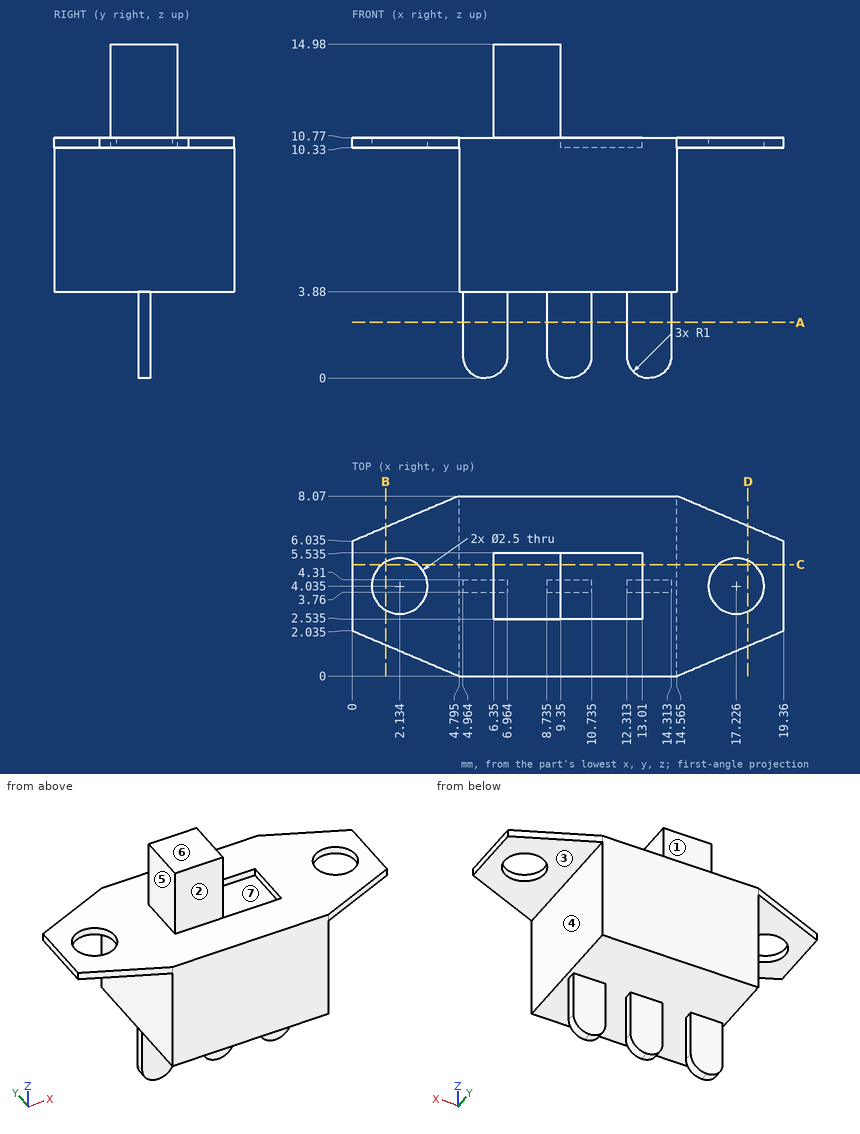
Verification items for this drawing (mm, ordinates from the low corner). A direction names the side the tool comes from. Round coordinates to 2 decimals unless told otherwise and drop trailing zeros. Write each loop counter-clockwise with the first axis right and the second up, starting at its lowest first coordinate (ties: lowest second). Pieces come first, ordered by that corner, then holes. Notation, with made-up numbers: (-20.75, 4.25) - (-4.75, 4.25) arc R31 ccw to (-4.75, 42.25) - close; hole circle Ø11 at (9, -19.75). An arc over 180 degrees is marked (long way). Answer as a JSON object with one key per item and string values. Group by question number.
Q1. Tool access check on the marked faces 1, 2 and 3. Record the directions out of +Z, -Z, +X, -X, +Y, -Y that give a thin tool (end or side, any length) a straight path to the whole face; none if there is none.
Q2. Thickness scan on line 1 (X direction, y = 2, z = 6.25) (1 decimal); line 2 (Z direction, x = 13.5, y = 0.75); line 3 (Z direction, x = 15.25, y = 3). Record the ranges inside material, lowest first.
Q3. Mould release check, pull along X, two halves, no side actions. Record for the marked faces 4, 5, 6 and 7: released by +X, released by -X, zero draft, split by the parting line, or undercut.
Q4. Go/stop test with flat-tipped pins: pin 1 Ø4 at (y, z) = (7, 8) entering from -X (1 decimal); pin 2 Ø3.5 at (x, y) = (12, 4.5) entering from +Z; pin 3 Ø1.6 at (x, z) = (14, 2) entering from +Y. Record where each tip stops, or that it passes through.
Q5. Section check A-A, the plane z = 2.5. Enter the section's corners in (x, y) (1 decimal).
Q6. Section check B-B, the plane x = 1.5. Enter the section's corners in (y, z).
Q7. Section check C-C, the plane y = 5. Give the number of separate pieces and of enclosed holes in the cut face.
Q8. Section check D-D, the plane x = 17.75. Enter the section's corners in (y, z).
Found:
{
 "1": {"face 1": "+Z, +X, -X, +Y", "face 2": "+Z, +X, -X, -Y", "face 3": "-Z, +X, +Y, -Y"},
 "2": {"line 1": "x = 4.8 to 14.6", "line 2": "z = 3.88 to 10.77", "line 3": "z = 10.33 to 10.77"},
 "3": {"face 4": "released by +X", "face 5": "released by -X", "face 6": "zero draft", "face 7": "undercut"},
 "4": {"pin 1": "stops at x = 4.8", "pin 2": "stops at z = 10.77", "pin 3": "stops at y = 4.31"},
 "5": {"outline": "(5, 3.8) - (7, 3.8) - (7, 4.3) - (5, 4.3) - close; (8.7, 3.8) - (10.7, 3.8) - (10.7, 4.3) - (8.7, 4.3) - close; (12.3, 3.8) - (14.3, 3.8) - (14.3, 4.3) - (12.3, 4.3) - close"},
 "6": {"outline": "(1.4, 10.33) - (2.96, 10.33) - (2.96, 10.77) - (1.4, 10.77) - close; (5.11, 10.33) - (6.67, 10.33) - (6.67, 10.77) - (5.11, 10.77) - close"},
 "7": {"separate pieces": "3", "enclosed holes": "0"},
 "8": {"outline": "(1.35, 10.33) - (2.9, 10.33) - (2.9, 10.77) - (1.35, 10.77) - close; (5.17, 10.33) - (6.72, 10.33) - (6.72, 10.77) - (5.17, 10.77) - close"}
}
